```python
from build123d import *

# Parameters (mm, degrees)
BOSS_EXTRUDE1_DEPTH             = 3.175
F_1_4_0_25_DIAMETER_HOLE1_D     = 6.35
F_1_4_0_25_DIAMETER_HOLE1_DEPTH = 9.268267535
F_1_4_0_25_DIAMETER_HOLE1_TIP   = 1.907732465
FILLET1_R                       = 12.7


with BuildPart() as part:
    # Sketch1 → Boss-Extrude1 (new body)
    with BuildSketch(Plane.XY):
        with BuildLine():
            Line((-26.289500227, -31.481815247), (-29.464500227, -31.481815247))
            Line((-29.464500227, -31.481815247), (-29.464500227, -12.431815247))
            Line((-29.464500227, -12.431815247), (-26.289500227, -12.431815247))
            Line((-26.289500227, -12.431815247), (-26.289500227, -6.081815247))
            Line((-26.289500227, -6.081815247), (-13.589500227, -6.081815247))
            Line((-13.589500227, -6.081815247), (8.000499773, -22.666158546))
            ThreePointArc((8.000499773, -22.666158546), (9.676721644, -37.516329042), (-3.937500227, -43.67995187))
            Line((-3.937500227, -43.67995187), (-26.289500227, -36.561815247))
            Line((-26.289500227, -36.561815247), (-26.289500227, -31.481815247))
        make_face()
    extrude(amount=BOSS_EXTRUDE1_DEPTH)

    # 1/4 (0.25) Diameter Hole1
    with Locations(Plane.XY.offset(3.175)):
        with Locations((-1.365750227, -31.243067134)):
            Hole(F_1_4_0_25_DIAMETER_HOLE1_D / 2, depth=F_1_4_0_25_DIAMETER_HOLE1_DEPTH)
            with Locations((0, 0, -(F_1_4_0_25_DIAMETER_HOLE1_DEPTH + F_1_4_0_25_DIAMETER_HOLE1_TIP / 2))):  # 118° drill point
                Cone(0, F_1_4_0_25_DIAMETER_HOLE1_D / 2, F_1_4_0_25_DIAMETER_HOLE1_TIP, mode=Mode.SUBTRACT)

    # Fillet1
    fillet1_edges = [part.edges().sort_by_distance(p)[0] for p in [
        (-13.589500227, -6.081815247, 1.5875),
    ]]
    fillet(fillet1_edges, radius=FILLET1_R)


solid = part.part
```
The model under review builds one solid part; all positions refer to its coordinate system, in mm. A direction names the side the tool comes from. Round coordinates to 2 decimals unless told otherwise and drop trailing zeros. Loops run counter-clockwise (first coordinate to the right, second up) from the corner with the lowest first, then second, coordinate; pieces in that order, holes last.
Item 1: Take a section at D-D (y = -15). Write out the cut boundary in (x, z) (1 decimal), then the cut area to 3 significant figures.
Determined:
outline: (-29.5, 0) - (-2, 0) - (-2, 3.2) - (-29.5, 3.2) - close
area: 87.3 mm2
Item 2: For faces 1 (the face through (-26.29, -9, 2)), 2 (the face through (-9, -25, 3.175)), 3 (the face through (-26.29, -34, 2)), list the 3-axis set-ups (+Z, -Z, +X, -X, +Y, -Y) from which the entire face can be reached by the end or side of a thin tool; tool diameter is ignored.
Determined:
face 1: +Z, -Z, -X, +Y
face 2: +Z, +X, -X, +Y, -Y
face 3: +Z, -Z, -X, -Y
Item 3: For line 1 (X direction, y = -30, z = 2.15); line 2 (X direction, y = -28.5, z = 0.6); line 3 (Y direction, x = 1.5, z = 2), list the stretches that pass through material, from the lowest coordinate up.
Determined:
line 1: x = -29.46 to -4.29, 1.56 to 11.27
line 2: x = -29.46 to -2.96, 0.23 to 11.03
line 3: y = -43.62 to -32.61, -29.88 to -17.67
Item 4: Mouldability with a two-part tool opening along Y and no side actions: class faces 4 (the face through (-28, -31.482, 2)), 5 (the face through (-9, -25, 0)), 6 (the face through (-22, -6.082, 2)), 7 (the face through (-0.952, -28.095, 1.565)) as released by +Y, released by -Y, zero draft, split by the parting line, or undercut.
Determined:
face 4: released by -Y
face 5: zero draft
face 6: released by +Y
face 7: undercut
Item 5: Clearance check with flat-ended pins moving along their axes: pin 1 Ø1 at (x, z) = (-28, 1.5) entering from -Y; pin 2 Ø8 at (x, y) = (-3.5, -32) entering from -Z; pin 3 Ø1.6 at (y, z) = (-34, 1.5) entering from -X. State where each tip first meets the part, or that it passes through.
Determined:
pin 1: stops at y = -31.48
pin 2: stops at z = 0
pin 3: stops at x = -26.29
Item 6: Take a section at C-C (x = -11). Write out the cut boundary in (y, z) (3 decimals), then the cut area to 3 significant figures.
Determined:
outline: (-41.431, 0) - (-8.122, 0) - (-8.122, 3.175) - (-41.431, 3.175) - close
area: 106 mm2
Item 7: Take a section at B-B (y = -30). Write out the cut boundary in (x, z) (1 decimal), then the cut area to 3 significant figures.
Determined:
outline: (-29.5, 0) - (-4.3, 0) - (-4.3, 3.2) - (-29.5, 3.2) - close; (1.6, 0) - (11.3, 0) - (11.3, 3.2) - (1.6, 3.2) - close
area: 111 mm2
